Can you work these out from the model? Positions are in its coordinate system, mm. Give positions to 0.01 mm unless a question says otherwise; leave off trailing zeros. Write each loop counter-clockwise with the first axis right and the second up, starting at its lowest first coordinate (ties: lowest second). Pieces come first, ordered by that corner, then holes. Notation, with made-up numbers: (-5, -18.75) - (22, -18.75) arc R25 cw to (22, 0.25) - close; hole circle Ø5 at (72.25, 41.25). An arc over 180 degrees is marked (long way). Use a Markdown table: item, result. Add a question column.
```python
from build123d import *

# Parameters (mm, degrees)
SKETCH_1_W               = 2600
SKETCH_1_H               = 600
EXTRUDE_1_DEPTH          = 38
FILLET_1_R               = 10
SKETCH_2_W               = 560
SKETCH_2_H               = 490
SKETCH_2_W_2             = 630
SKETCH_2_H_2             = 475
CUT_EXTRUDE_1_DEPTH      = 1
CUT_EXTRUDE_1_DEPTH_BACK = 39


with BuildPart() as part:
    # Эскиз1 → Бобышка-Вытянуть1 (new body)
    with BuildSketch(Plane(origin=(0, 0, 0), x_dir=(1, 0, 0), z_dir=(0, 1, 0))):
        Rectangle(SKETCH_1_W, SKETCH_1_H)
    extrude(amount=EXTRUDE_1_DEPTH)

    # Скругление1
    fillet_1_edges = [part.edges().sort_by_distance(p)[0] for p in [
        (0, 0, 300),
        (0, 38, 300),
    ]]
    fillet(fillet_1_edges, radius=FILLET_1_R)

    # Эскиз2 → Вырез-Вытянуть1 (cut, two sides)
    with BuildSketch(Plane(origin=(0, 38, 0), x_dir=(1, 0, 0), z_dir=(0, 1, 0))) as cut_extrude_1_sk:
        with Locations((-120, -5)):
            Rectangle(SKETCH_2_W, SKETCH_2_H)
        with Locations((-946, 0)):
            Rectangle(SKETCH_2_W_2, SKETCH_2_H_2)
    extrude(amount=CUT_EXTRUDE_1_DEPTH, mode=Mode.SUBTRACT)
    extrude(cut_extrude_1_sk.sketch, amount=-CUT_EXTRUDE_1_DEPTH_BACK, mode=Mode.SUBTRACT)


solid = part.part
```
Q1. Suppose I cut it at D-D (x = -1070). Please give me the cut outline in (y, z), and give its area (3 significant figures).
Q2. If I drill on probe 1 along X at (y, z) = (24, -159); probe 2 along Z at (x, y) = (-765.5, 12); probe 3 along Z at (x, y) = (55, 10), over which ranges is the centre line in solid material (lowest first)? Write a range as [from, to].
Q3. Suppose I cut it at A-A (x = -229). Please give me the cut outline in (y, z).
Q4. I'm going to push a flat-ended pin straight in: P1, Ø4, axis at x = 468.5, y = 8.5, coming from the +Z side. Where does the tip first touch, or does it pass through?
Q5. Suppose I cut it at C-C (y = 22). Please give me the cut outline in (x, z).
Q6. Suppose I cut it at B-B (z = 58.5). Please give me the cut outline in (x, y), and give its area (3 significant figures).
Derived:
| question | item | result |
|---|---|---|
| 1 | outline | (0, -300) - (38, -300) - (38, -237.5) - (0, -237.5) - close; (0, 237.5) - (38, 237.5) - (38, 290) arc R10 ccw to (28, 300) - (10, 300) arc R10 ccw to (0, 290) - close |
| 1 | area | 4,710 mm² |
| 2 | probe 1 | [-1300, -1261], [-631, -400], [160, 1300] |
| 2 | probe 2 | [-300, -237.5], [237.5, 300] |
| 2 | probe 3 | [-300, -240], [250, 300] |
| 3 | outline | (0, -300) - (38, -300) - (38, -240) - (0, -240) - close; (0, 250) - (38, 250) - (38, 290) arc R10 ccw to (28, 300) - (10, 300) arc R10 ccw to (0, 290) - close |
| 4 | P1 | z = 300 |
| 5 | outline | (-1300, -300) - (1300, -300) - (1300, 300) - (-1300, 300) - close; hole (-1261, -237.5) - (-631, -237.5) - (-631, 237.5) - (-1261, 237.5) - close; hole (-400, -240) - (160, -240) - (160, 250) - (-400, 250) - close |
| 6 | outline | (-1300, 0) - (-1261, 0) - (-1261, 38) - (-1300, 38) - close; (-631, 0) - (-400, 0) - (-400, 38) - (-631, 38) - close; (160, 0) - (1300, 0) - (1300, 38) - (160, 38) - close |
| 6 | area | 53,600 mm² |
